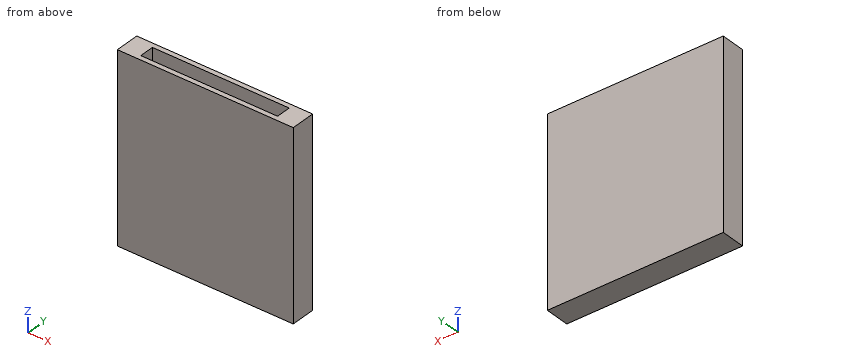
Autodesk Inventor part; units mm, degrees
ref_plane "YZ Plane" through (0, 0, 0) normal (1, 0, 0) x (0, 1, 0)
ref_plane "XZ Plane" through (0, 0, 0) normal (0, 1, 0) x (-1, 0, 0)
ref_plane "XY Plane" through (0, 0, 0) normal (0, 0, 1) x (1, 0, 0)
sketch "Sketch2" plane through (0, 0, 0) normal (0, 0, 1) x (1, 0, 0)
  line L0 (-7.2, 1) -> (7.2, 1)
  line L1 (7.2, 1) -> (7.2, -1)
  line L2 (7.2, -1) -> (-7.2, -1)
  line L3 (-7.2, -1) -> (-7.2, 1)
  line L4 (-5.6, 0.6) -> (5.6, 0.6)
  line L5 (5.6, 0.6) -> (5.6, -0.6)
  line L6 (5.6, -0.6) -> (-5.6, -0.6)
  line L7 (-5.6, -0.6) -> (-5.6, 0.6)
  point P0 (0, 0)
  point P1 (-7.2, 0)
  point P2 (0, -1)
  point P3 (0, 0.6)
  point P4 (-5.6, 0)
  dimension "d0" = 2
  dimension "d1" = 14.4
  dimension "d2" = 1.2
  dimension "d3" = 11.2
extrude "Extrusion1" add sketch "Sketch2" against normal blind 15.2 contours L0 L1 L2 L3 | L4 L5 L6 L7
extrude "Extrusion2" cut sketch "Sketch2" against normal blind 14.4 contours L4 L5 L6 L7
properties part number "11034-Black" material "ABS Plastic"
Here's how the part is built. I have some questions about the finished solid (model axes, mm). Coordinates: 2 decimals unless noted, no trailing zeros. Write each loop counter-clockwise with the first axis right and the second up, starting at its lowest first coordinate (ties: lowest second). Pieces come first, ordered by that corner, then holes.
Item 1: I want a section at C-C on x = -3.75. Write out the boundary of the cut face in (y, z).
Item 2: I want a section at B-B on y = 0.05. Write out the boundary of the cut face in (x, z).
Item 3: I want a section at A-A on z = -2.25. Write out the boundary of the cut face in (x, y), and give its area (3 significant figures).
Item 4: If I drill on line 1 (Y direction, x = -1.5, z = -2); line 2 (X direction, y = -0.45, z = -7.5); line 3 (Z direction, x = 4.5, y = 0.5), over which ranges is the centre line in solid material (lowest first)?
Findings below:
1. outline: (-1, -15.2) - (1, -15.2) - (1, 0) - (0.6, 0) - (0.6, -14.4) - (-0.6, -14.4) - (-0.6, 0) - (-1, 0) - close
2. outline: (-7.2, -15.2) - (7.2, -15.2) - (7.2, 0) - (5.6, 0) - (5.6, -14.4) - (-5.6, -14.4) - (-5.6, 0) - (-7.2, 0) - close
3. outline: (-7.2, -1) - (7.2, -1) - (7.2, 1) - (-7.2, 1) - close; hole (-5.6, -0.6) - (5.6, -0.6) - (5.6, 0.6) - (-5.6, 0.6) - close
3. area: 15.4 mm2
4. line 1: y = -1 to -0.6, 0.6 to 1
4. line 2: x = -7.2 to -5.6, 5.6 to 7.2
4. line 3: z = -15.2 to -14.4
